Could you check a few things on this drawing? It's one solid part, dimensions in mm from its lowest x, y, z. Coordinates: 2 decimals unless noted, no trailing zeros. Order: outer loops, then holes, each group sorted by start corner. A loop starts at its lowest first (then second) coordinate and runs counter-clockwise, first axis right, second up. Notation, with made-up numbers: (-23.5, 35) - (33.5, 35) arc R25 cw to (33.5, 53) - close; hole circle Ø9 at (59, 89). An arc over 180 degrees is marked (long way). Answer in a Markdown table with one row per item. Add a question column.
Item 1: If I drill on line 1 along Y through (x, z) = (25, 35); line 2 along Z through (x, y) = (37.5, 9); line 3 along Y through (x, z) = (20.5, 46), over which ranges is the centre line in solid material (lowest first)? Write a range as from..to.
Item 2: Thinking about a two-plate mould opening in Y: for the marked faces 1, 2 and 3, which applies, +Y half, -Y half, draft (parallel to the pull), parting line (faces both ways), or undercut?
Item 3: Will these pins go through, and if not, where does the flat tip stop? pin 1 Ø8 at (y, z) = (36.5, 30) entering from -X; pin 2 Ø6 at (x, z) = (14.5, 48.5) entering from -Y; pin 3 Ø5 at (x, z) = (44, 29) entering from -Y.
Item 4: I want a section at B-B (z = 8.5). Please give me the cut outline in (x, y), plus the area to 3 significant figures.
Item 5: I want a section at A-A (z = 52.5). Please give me the cut outline in (x, y).
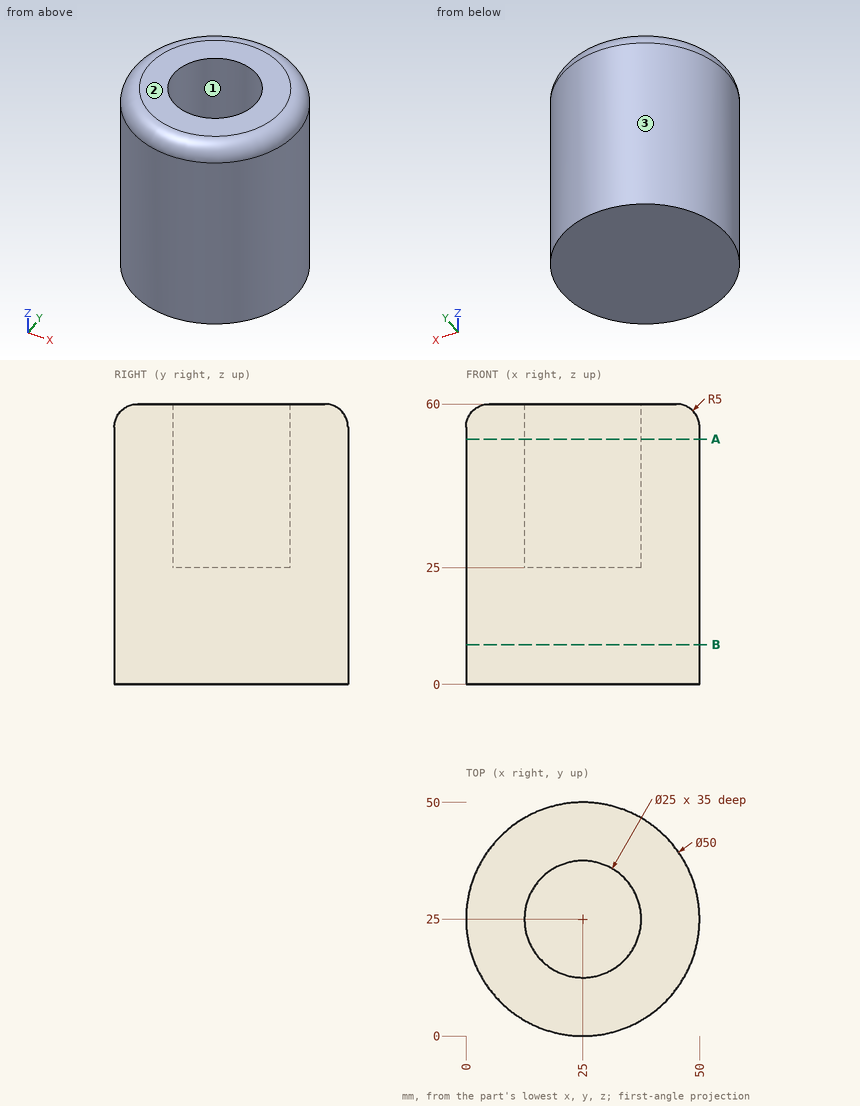
Values follow:
| question | item | result |
|---|---|---|
| 1 | line 1 | y = 0..12.5, 37.5..50 |
| 1 | line 2 | z = 0..59.99 |
| 1 | line 3 | y = 0.41..13.34, 36.66..49.59 |
| 2 | face 1 | undercut |
| 2 | face 2 | draft |
| 2 | face 3 | parting line |
| 3 | pin 1 | stops at x = 1.15 |
| 3 | pin 2 | stops at y = 1.15 |
| 3 | pin 3 | stops at y = 6.22 |
| 4 | outline | circle Ø50 at (25, 25) |
| 4 | area | 1,960 mm^2 |
| 5 | outline | circle Ø50 at (25, 25); hole circle Ø25 at (25, 25) |
